Design review of the part shown in the three views and the two pictorial views. Dimensions are in mm from the part's minimum x, y and z. Give positions to 0.01 mm unless a question says otherwise; leave off trailing zeros. Order: outer loops, then holes, each group sorted by start corner. A loop starts at its lowest first (then second) coordinate and runs counter-clockwise, first axis right, second up. Notation, with made-up numbers: M -33.75,84 L -8.75,84 A21 ccw -8.75,119 Z; hole C -31.5,15 d7. An arc over 180 degrees is marked long. Answer as a JSON object with one key per item and string values.
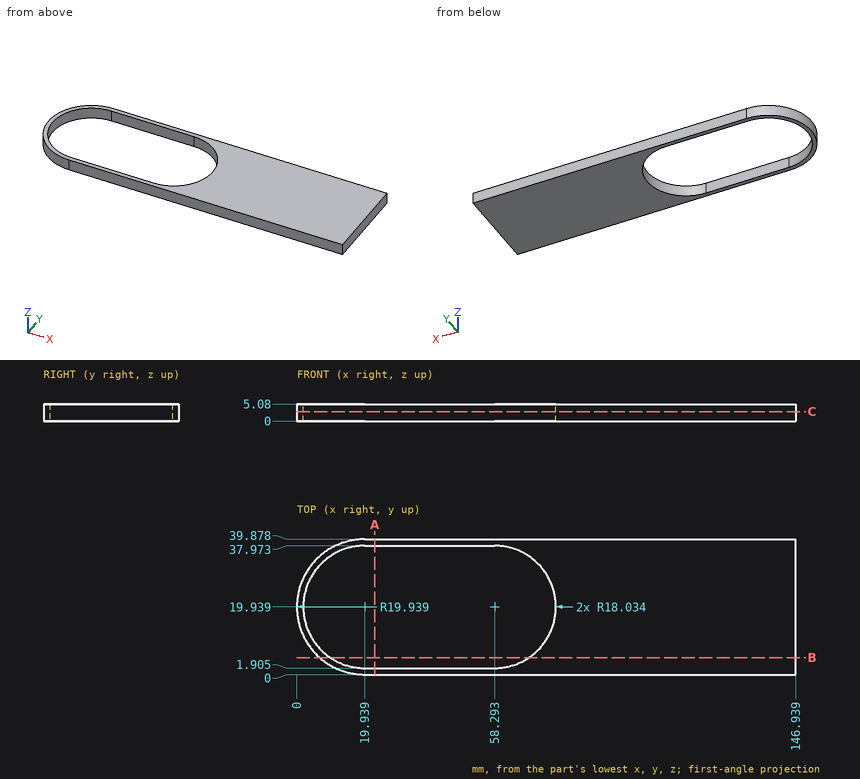
(1) We need section B-B (y = 5). Write out the cut boundary in (x, z), plus the area to 3 significant figures.
Checked values:
{"outline": "M 6.73,0 L 9.84,0 L 9.84,5.08 L 6.73,5.08 Z; M 68.4,0 L 146.94,0 L 146.94,5.08 L 68.4,5.08 Z", "area": "415 mm^2"}
(2) We need section C-C (z = 2.8). Write out the cut boundary in (x, y) (3 decimals).
Checked values:
{"outline": "M 19.939,0 L 146.939,0 L 146.939,39.878 L 19.939,39.878 A19.939 ccw Z; hole M 19.939,1.905 L 58.293,1.905 A18.034 ccw 58.293,37.973 L 19.939,37.973 A18.034 ccw Z"}
(3) To check wall thickness, follow L1, parallel to Y at x = 33, z = 1.9 (3 decimals); L2, parallel to X at y = 20.5, z = 3.8; L3, parallel to X at y = 10, z = 2.5. State the ranges of each line that lie inside material, in increasing order. Write a range as from..to.
Checked values:
{"L1": "y = 0..1.905, 37.973..39.878", "L2": "x = 0.01..1.91, 76.32..146.94", "L3": "x = 2.65..4.89, 73.34..146.94"}
(4) We need section A-A (x = 23). Write out the cut boundary in (y, z) (3 decimals).
Checked values:
{"outline": "M 0,0 L 1.905,0 L 1.905,5.08 L 0,5.08 Z; M 37.973,0 L 39.878,0 L 39.878,5.08 L 37.973,5.08 Z"}
(5) Insertion check: pin 1 (2 mm diameter, centred on y = 22.5, z = 1, fed in from -X). The pin has a flat end and moves straight along its axis. Give the tip position at first contact, or say it passes through.
Checked values:
{"pin 1": "stops at x = 0.06"}
